from build123d import *

# Parameters (mm, degrees)
BOSS_EXTRUDE1_DEPTH = 1016


with BuildPart() as part:
    # Sketch1 → Boss-Extrude1 (new body)
    with BuildSketch(Plane(origin=(0, 0, 0), x_dir=(1, 0, 0), z_dir=(0, 1, 0))):
        Polygon((0, 1016), (0, 508), (1524, 0), (1524, 508), align=None)
        Polygon((1524, 1016), (0, 1016), (1524, 508), align=None)
        Polygon((0, 508), (0, 0), (1524, 0), align=None)
    extrude(amount=BOSS_EXTRUDE1_DEPTH)

    # SurfaceCut1
    split(bisect_by=Plane(origin=(320.842105263, 962.526315789, -962.526315789), x_dir=(-0.9733285267845753, 0.16222142113076252, -0.1622214211307626), z_dir=(0.22941573387056174, 0.6882472016116851, -0.6882472016116855)), keep=Keep.BOTTOM)

    # SurfaceCut2
    split(bisect_by=Plane(origin=(-80.210526316, 240.631578947, 240.631578947), x_dir=(0.9733285267845753, 0.16222142113076254, 0.16222142113076254), z_dir=(-0.22941573387056177, 0.6882472016116853, 0.6882472016116854)), keep=Keep.BOTTOM)


solid = part.part
Geometry check sheet. Reference: the model listing, model coordinates, mm. Give positions to 0.01 mm unless a question says otherwise; leave off trailing zeros. Order: outer loops, then holes, each group sorted by start corner. A loop starts at its lowest first (then second) coordinate and runs counter-clockwise, first axis right, second up. Notation, with made-up numbers: M -21,60.5 L -7,60.5 A22 cw -7,72.5 Z; hole C 54.25,80 d6. An arc over 180 degrees is marked long. Use a Markdown table: item, result.
Item 1: Section check A-A (z = -179.5). Record the cut outline in (x, y), and give its area (3 significant figures).
Answers follow:
| item | result |
|---|---|
| outline | M 0,0 L 1524,0 L 1524,1016 L 985.5,1016 L 0,687.5 Z |
| area | 1,390,000 mm2 |
Item 2: Material ranges on line 1 along Y through (x, z) = (489, -881); line 2 along Z through (x, y) = (882.5, 952); line 3 along Y through (x, z) = (501.5, -320.5), recorded low to high.
Answers follow:
| item | result |
|---|---|
| line 1 | y = 0 to 988 |
| line 2 | z = -785.83 to -149.83 |
| line 3 | y = 0 to 995.67 |
Item 3: Section check C-C (x = 114). Record the cut outline in (y, z), and give its area (3 significant figures).
Answers follow:
| item | result |
|---|---|
| outline | M 0,-1016 L 978,-1016 L 1016,-978 L 1016,-470 L 546,0 L 0,0 Z |
| area | 921,000 mm2 |
Item 4: Section check D-D (z = -355.5). Record the cut outline in (x, y), and give its area (3 significant figures).
Answers follow:
| item | result |
|---|---|
| outline | M 0,0 L 1524,0 L 1524,1016 L 457.5,1016 L 0,863.5 Z |
| area | 1,510,000 mm2 |
Item 5: Section check B-B (y = 815). Record the cut outline in (x, z).
Answers follow:
| item | result |
|---|---|
| outline | M 0,-1016 L 603,-1016 L 1524,-709 L 1524,0 L 921,0 L 0,-307 Z |
